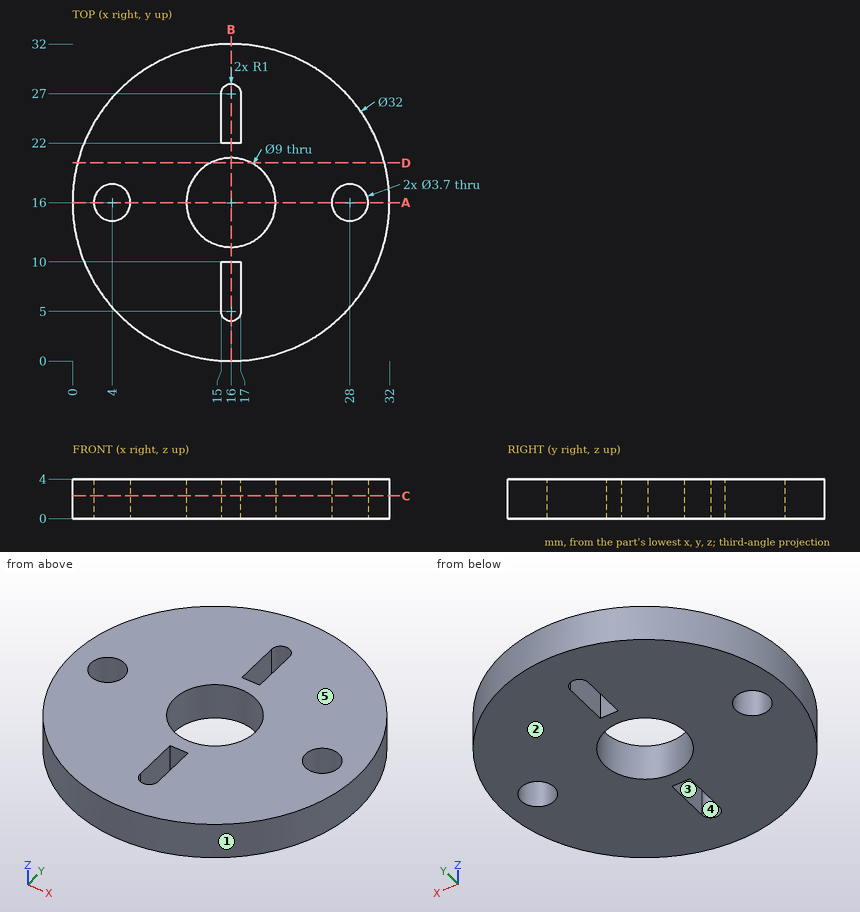
Could you check a few things on this drawing? It's one solid part, dimensions in mm from its lowest x, y, z. A direction names the side the tool comes from. Give positions to 0.01 mm unless a question says otherwise; leave off trailing zeros. Loops run counter-clockwise (first coordinate to the right, second up) from the corner with the lowest first, then second, coordinate; pieces in that order, holes last. Notation, with made-up numbers: M 48.5,51 L 79.5,51 A17 cw 79.5,68 Z; hole C -33,28.25 d5. An arc over 180 degrees is marked long. Answer as a JSON object with one key per item and string values.
Q1. Suppose I cut it at D-D, the plane y = 20. List the corners of the cut face in (x, z) for me.
Values found:
{"outline": "M 0.51,0 L 13.94,0 L 13.94,4 L 0.51,4 Z; M 18.06,0 L 31.49,0 L 31.49,4 L 18.06,4 Z"}
Q2. Suppose I cut it at B-B, the plane x = 16. List the corners of the cut face in (y, z) for me.
Values found:
{"outline": "M 0,0 L 4,0 L 4,4 L 0,4 Z; M 10,0 L 11.5,0 L 11.5,4 L 10,4 Z; M 20.5,0 L 22,0 L 22,4 L 20.5,4 Z; M 28,0 L 32,0 L 32,4 L 28,4 Z"}
Q3. For the marked faces 4 and 5, which set-ups out of +Z, -Z, +X, -X, +Y, -Y let a thin tool reach every point of the face, with its end or its side?
Values found:
{"face 4": "+Z, -Z", "face 5": "+Z, +X, -X, +Y, -Y"}
Q4. If I drill on probe 1 along X at (y, z) = (6, 2.75); probe 2 along Y at (x, z) = (12, 3.8); probe 3 along Y at (x, z) = (4.5, 0.3), over which ranges is the centre line in solid material (lowest first)? Write a range as [from, to].
Values found:
{"probe 1": "x = [3.51, 15], [17, 28.49]", "probe 2": "y = [0.51, 13.94], [18.06, 31.49]", "probe 3": "y = [4.88, 14.22], [17.78, 27.12]"}
Q5. Suppose I cut it at C-C, the plane z = 2.3. List the corners of the cut face in (x, y) for me, plus the area to 3 significant figures.
Values found:
{"outline": "C 16,16 d32; hole C 4,16 d3.7; hole C 16,16 d9; hole M 15,5 A1 ccw 17,5 L 17,10 L 15,10 Z; hole M 15,22 L 17,22 L 17,27 A1 ccw 15,27 Z; hole C 28,16 d3.7", "area": "696 mm²"}
Q6. For P1, Ø2, axis at x = 4, y = 16, coming from the +Z side; P2, Ø1, axis at y = 21, z = 2.5, coming from the -X side; P3, Ø2, axis at y = 7, z = 2.5, coming from the -X side; P4, Ø1, axis at y = 21.5, z = 1, coming from the -X side, each with a flat end and sliding along its axis, tell me the tip position at first contact or that it passes through.
Values found:
{"P1": "passes through", "P2": "stops at x = 0.65", "P3": "stops at x = 2.14", "P4": "stops at x = 0.8"}
Q7. If we mould it in two halves opening along X, with no side actions, what happens to the marked faces 1, 2 and 3? For each: pulls with the +X half, pulls with the -X half, needs draft (parallel to the pull), parting line crosses it, or undercut.
Values found:
{"face 1": "parting line crosses it", "face 2": "needs draft", "face 3": "undercut"}
Q8. Suppose I cut it at A-A, the plane y = 16. List the corners of the cut face in (x, z) for me.
Values found:
{"outline": "M 0,0 L 2.15,0 L 2.15,4 L 0,4 Z; M 5.85,0 L 11.5,0 L 11.5,4 L 5.85,4 Z; M 20.5,0 L 26.15,0 L 26.15,4 L 20.5,4 Z; M 29.85,0 L 32,0 L 32,4 L 29.85,4 Z"}
